Model file for the job. Use its own axes, mm. A direction names the side the tool comes from. Coordinates: 2 decimals unless noted, no trailing zeros. Write each loop counter-clockwise with the first axis right and the second up, starting at its lowest first coordinate (ties: lowest second). Pieces come first, ordered by that corner, then holes.
Q1. Pull direction X, two halves, no side cores. Call faces 5 (the flat face through (57.5, -81, 1)), 6 (the cylindrical face through (41.61, -43.14, 10.1)), 7 (the flat face through (34.8, -59.9, 3)), 8 (the flat face through (52.91, -47.48, 8.5)): released by +X, released by -X, zero draft, split by the parting line, or undercut.
Q2. Band-saw the part on A-A, the plane z = 7.25. Write the cut outline in (x, y).
Q3. Drill centre lines: probe 1 along X at (y, z) = (-64, 12.5); probe 2 along X at (y, z) = (-45, 16.5); probe 3 along Y at (x, z) = (65, 5.75). Where is each one in solid material? Low to high.
Q4. Which spindle directions (+Z, -Z, +X, -X, +Y, -Y) get a long thin tool onto all of the face, cutting with end or side? Do faces 1 (the flat face through (76, -60, 0)), 2 (the flat face through (75.875, -60, 18)), 3 (the flat face through (62.5, -39, 1)), 4 (the flat face through (45.612, -60, 9)). Say none if no direction does.
Q5. Pin check, flat tips, straight feed: P1, Ø1, axis at y = -68.5, z = 4, coming from the +X side; P2, Ø2, axis at y = -38.5, z = 1.5, coming from the +X side; P3, Ø0.8, axis at y = -81.5, z = 1.5, coming from the -X side. Stop position of each tip, or through.
from build123d import *

# Parameters (mm, degrees)
POCKET025_DEPTH      = 19.001
POCKET026_DEPTH      = 1.25
CHAMFER002_SIZE      = 2
CHAMFER003_SIZE      = 0.5
POCKET027_DEPTH      = 28.501
POCKET027_DEPTH_BACK = 28.501


with BuildPart() as part:
    # Sketch035 (on XZ_Plane051 of Origin104) → Revolution011 (revolve)
    with BuildSketch(Plane.XZ):
        Polygon((0, 0), (24.95, 0), (28.5, 3), (24.95, 3), (24.95, 19), (0, 19), align=None)
    revolve(axis=Axis((0, 0, 0), (0, 0, 1)))

    # Sketch036 (on XY_Plane051 of Origin104) → Pocket025 (cut, through all)
    with BuildSketch(Plane.XY):
        Polygon((14.3875, 8.306627), (0, 16.613254), (-14.3875, 8.306627), (-14.3875, -8.306627), (0, -16.613254), (14.3875, -8.306627), align=None)
    extrude(amount=POCKET025_DEPTH, mode=Mode.SUBTRACT)

    # Sketch037 (on XY_Plane051 of Origin104) → Pocket026 (cut)
    with BuildSketch(Plane.XY.offset(19)):
        Polygon((15.875, -9.165436), (15.875, 9.165436), (0, 18.330871), (-15.875, 9.165436), (-15.875, -9.165436), (0, -18.330871), align=None)
    extrude(amount=-POCKET026_DEPTH, mode=Mode.SUBTRACT)

    # Chamfer002
    chamfer002_edges = [part.edges().sort_by_distance(p)[0] for p in [
        (-24.95, 0, 19),
    ]]
    chamfer(chamfer002_edges, length=CHAMFER002_SIZE)

    # Chamfer003
    chamfer003_edges = [part.edges().sort_by_distance(p)[0] for p in [
        (-14.3875, 0, 17.75),
        (-7.19375, 12.45994, 17.75),
        (7.19375, 12.45994, 17.75),
        (14.3875, 0, 17.75),
        (7.19375, -12.45994, 17.75),
        (-7.19375, -12.45994, 17.75),
    ]]
    chamfer(chamfer003_edges, length=CHAMFER003_SIZE)

    # Sketch038 (on XZ_Plane052 of Origin104) → Pocket027 (cut, two sides)
    with BuildSketch(Plane.XZ) as pocket027_sk:
        with BuildLine():
            ThreePointArc((2.5, 2.5), (0, 5), (-2.5, 2.5))
            Line((-2.5, 2.5), (-2.5, -2.5))
            Line((-2.5, -2.5), (2.5, -2.5))
            Line((2.5, -2.5), (2.5, 2.5))
        make_face()
    extrude(amount=-POCKET027_DEPTH, mode=Mode.SUBTRACT)
    extrude(pocket027_sk.sketch, amount=POCKET027_DEPTH_BACK, mode=Mode.SUBTRACT)


with BuildPart() as part_1:
    # Body056 placement: moved
    add(part.part.moved(Location((60, -60, 0))))


solid = part_1.part
Answer sheet:
1. face 5: undercut
1. face 6: split by the parting line
1. face 7: zero draft
1. face 8: undercut
2. outline: circle Ø49.9 at (60, -60); hole (45.61, -68.31) - (60, -76.61) - (74.39, -68.31) - (74.39, -51.69) - (60, -43.39) - (45.61, -51.69) - close
3. probe 1: x = 35.37 to 45.61, 74.39 to 84.63
3. probe 2: x = 40.06 to 57.21, 62.79 to 79.94
3. probe 3: y = -84.44 to -73.73, -46.27 to -35.56
4. face 1: -Z, +X, -X, +Y, -Y
4. face 2: +Z
4. face 3: -Z, +Y, -Y
4. face 4: +Z, -Z
5. P1: stops at x = 83.63
5. P2: stops at x = 78.14
5. P3: stops at x = 43.19
